```python
from build123d import *

# Parameters (mm, degrees)
SKETCH1_W           = 36.576
SKETCH1_H           = 36.576
BOSS_EXTRUDE1_DEPTH = 2.54
SKETCH2_R           = 0.889
BOSS_EXTRUDE2_DEPTH = 25.4
CUT_EXTRUDE4_DEPTH  = 3.54
SKETCH4_R           = 8.001
BOSS_EXTRUDE3_DEPTH = 1.016
SKETCH5_R           = 2.49555
BOSS_EXTRUDE4_DEPTH = 19.05
SKETCH6_R           = 18.161
BOSS_EXTRUDE5_DEPTH = 20.828


with BuildPart() as part:
    # Sketch1 → Boss-Extrude1 (new body)
    with BuildSketch(Plane.XY):
        with Locations((17.649916168, -17.343808383)):
            Rectangle(SKETCH1_W, SKETCH1_H)
    extrude(amount=BOSS_EXTRUDE1_DEPTH)

    # Sketch2 → Boss-Extrude2 (add)
    with BuildSketch(Plane.XY.offset(2.54)):
        with Locations((33.143916168, -1.849808383)):
            Circle(SKETCH2_R)
        with Locations((2.155916168, -32.837808383)):
            Circle(SKETCH2_R)
    extrude(amount=BOSS_EXTRUDE2_DEPTH)

    # Sketch3 → Cut-Extrude4 (cut, through all)
    with BuildSketch(Plane.XY.offset(2.54)):
        with BuildLine():
            Line((-0.638083832, 0.944191617), (-0.638083832, -17.343808383))
            Line((-0.638083832, -17.343808383), (-0.511083832, -17.343808383))
            ThreePointArc((-0.511083832, -17.343808383), (4.808149915, -4.50204213), (17.649916168, 0.817191617))
            Line((17.649916168, 0.817191617), (17.649916168, 0.944191617))
            Line((17.649916168, 0.944191617), (-0.638083832, 0.944191617))
        make_face()
        with BuildLine():
            Line((35.937916168, -35.631808383), (17.649916168, -35.631808383))
            Line((17.649916168, -35.631808383), (17.649916168, -35.504808383))
            ThreePointArc((17.649916168, -35.504808383), (30.491682421, -30.185574636), (35.810916168, -17.343808383))
            Line((35.810916168, -17.343808383), (35.937916168, -17.343808383))
            Line((35.937916168, -17.343808383), (35.937916168, -35.631808383))
        make_face()
    extrude(amount=-CUT_EXTRUDE4_DEPTH, mode=Mode.SUBTRACT)

    # Sketch4 → Boss-Extrude3 (add)
    with BuildSketch(Plane(origin=(0, 0, 0), x_dir=(-1, 0, 0), z_dir=(0, 0, -1))):
        with Locations((-17.649916168, -17.343808383)):
            Circle(SKETCH4_R)
    extrude(amount=BOSS_EXTRUDE3_DEPTH)

    # Sketch5 → Boss-Extrude4 (add)
    with BuildSketch(Plane(origin=(0, 0, -1.016), x_dir=(-1, 0, 0), z_dir=(0, 0, -1))):
        with Locations((-17.649916168, -17.343808383)):
            Circle(SKETCH5_R)
    extrude(amount=BOSS_EXTRUDE4_DEPTH)

    # Sketch6 → Boss-Extrude5 (add)
    with BuildSketch(Plane.XY.offset(2.54)):
        with Locations((17.649916168, -17.343808383)):
            Circle(SKETCH6_R)
    extrude(amount=BOSS_EXTRUDE5_DEPTH)


solid = part.part
```
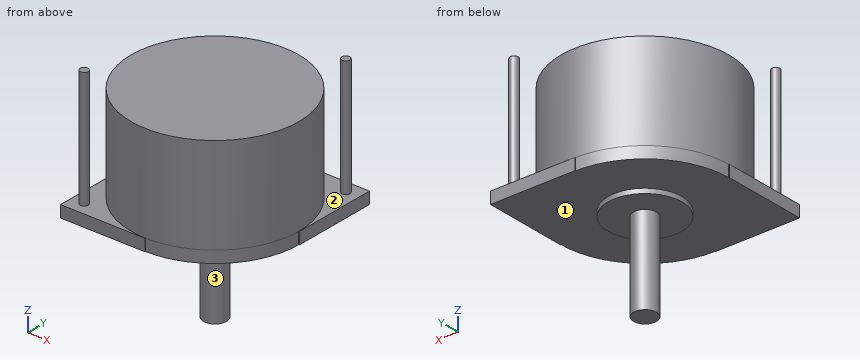
Part model, mm, in its own coordinate system. Face numbers are marked on the shaded views. Round coordinates to 2 decimals unless told otherwise and drop trailing zeros. Write each loop counter-clockwise with the first axis right and the second up, starting at its lowest first coordinate (ties: lowest second). Pieces come first, ordered by that corner, then holes. Notation, with made-up numbers: M 37.25,0.5 L 73.25,0.5 A20 cw 73.25,32.5 Z; hole C -6.5,78.5 d9. An arc over 180 degrees is marked long. Answer as CSV lines item,"result". Start each with the question number.
1) Mould opens along X. For the marked faces 1, 2 and 3 say: +X half, -X half, draft (parallel to the pull), parting line (faces both ways), or undercut.
2) Band-saw the part on C-C (z = -5.5). List the corners of the cut face in (x, y), then the cut area to 3 significant figures.
3) Drill centre lines: L1, parallel to Z at x = 25, y = -0.5; L2, parallel to Z at x = 27.5, y = -28; L3, parallel to Y at x = 33.5, z = 16. Where is each one in solid material? Low to high.
4) Band-saw the part on A-A (x = 6). List the corners of the cut face in (y, z), then the cut area to 3 significant figures.
5) Band-saw the part on B-B (y = -8). List the corners of the cut face in (x, z), then the cut area to 3 significant figures.
6) Band-saw the part on D-D (z = 17). List the corners of the cut face in (x, y), then the cut area to 3 significant figures.
7) Drop flat-ended pins along their axis: pin 1 (6 mm diameter, centred on x = 15, z = -9.5, fed in from +Y); pin 2 (10 mm diameter, centred on x = 30.5, y = -19, fed in from -Z); pin 3 (5 mm diameter, centred on x = 28.5, z = 15, fed in from -Y); pin 4 (18.5 mm diameter, centred on x = 16.5, y = -11.5, fed in from -Z). Give the stop position or say it passes through.
Worked out:
1,face 1,"draft"
1,face 2,"undercut"
1,face 3,"parting line"
2,outline,"C 17.65,-17.34 d4.99"
2,area,"19.6 mm²"
3,L1,"0 to 2.54"
3,L2,"0 to 23.37"
3,L3,"-26.21 to -8.48, -2.66 to -1.04"
4,outline,"M -35.63,0 L -3.41,0 L -3.41,23.37 L -31.28,23.37 L -31.28,2.54 L -35.63,2.54 Z"
4,area,"662 mm²"
5,outline,"M 2.08,0 L 35.94,0 L 35.94,2.54 L 33.22,2.54 L 33.22,23.37 L 2.08,23.37 Z"
5,area,"735 mm²"
6,outline,"C 17.65,-17.34 d36.32; C 2.16,-32.84 d1.78; C 33.14,-1.85 d1.78"
6,area,"1,040 mm²"
7,pin 1,"y = -14.85"
7,pin 2,"z = -1.02"
7,pin 3,"y = -33.47"
7,pin 4,"z = -20.07"
